Input: dimensioned drawing with shaded views. Units: mm. Origin: part minimum x, y, z. A direction names the side the tool comes from. Coordinates: 2 decimals unless noted, no trailing zeros. Order: outer loops, then holes, each group sorted by start corner. A loop starts at its lowest first (then second) coordinate and runs counter-clockwise, first axis right, second up. Notation, with made-up numbers: (-9.5, -13) - (5.5, -13) arc R25 ccw to (5.5, 20) - close; hole circle Ø5 at (32.5, 29.25). An arc over 180 degrees is marked (long way). One line per question, with ' | ' between items. Start each with the question number.
(1) Section A-A (x = 31.5). Return the cut outline in (y, z), then the cut area to 3 significant figures.
(2) Line query: line 1 along X through (y, z) = (5, 19); line 2 along Z through (x, y) = (62, 10); line 3 along X through (y, z) = (60.5, 26). Output: solid intervals per line, ascending.
(3) Contact query for flat-ended pins moving along their axis: P1, Ø8, axis at x = 10, y = 68.5, coming from the +Z side; P2, Ø12, axis at y = 37.5, z = 19.5, coming from the +X side; P3, Ø17.5, axis at x = 54.5, y = 65.5, coming from the +Z side. Output: stop coordinate, or through.
(4) Access query for the marked faces 1 and 2. Directions: +Z, -Z, +X, -X, +Y, -Y. A direction counts if a zero-diameter tool reaches every point of the face in a straight line with its end or side. Return the directions, or none.
(5) Draft query along Z for the marked faces 3, 4, 5 and 6. Return one class per face: +Z half, -Z half, draft (parallel to the pull), parting line (faces both ways), or undercut.
(6) Section D-D (x = 49). Return the cut outline in (y, z).
(7) Section C-C (z = 20.5). Return the cut outline in (x, y), then the cut area to 3 significant figures.
(8) Section B-B (y = 21). Return the cut outline in (x, z).
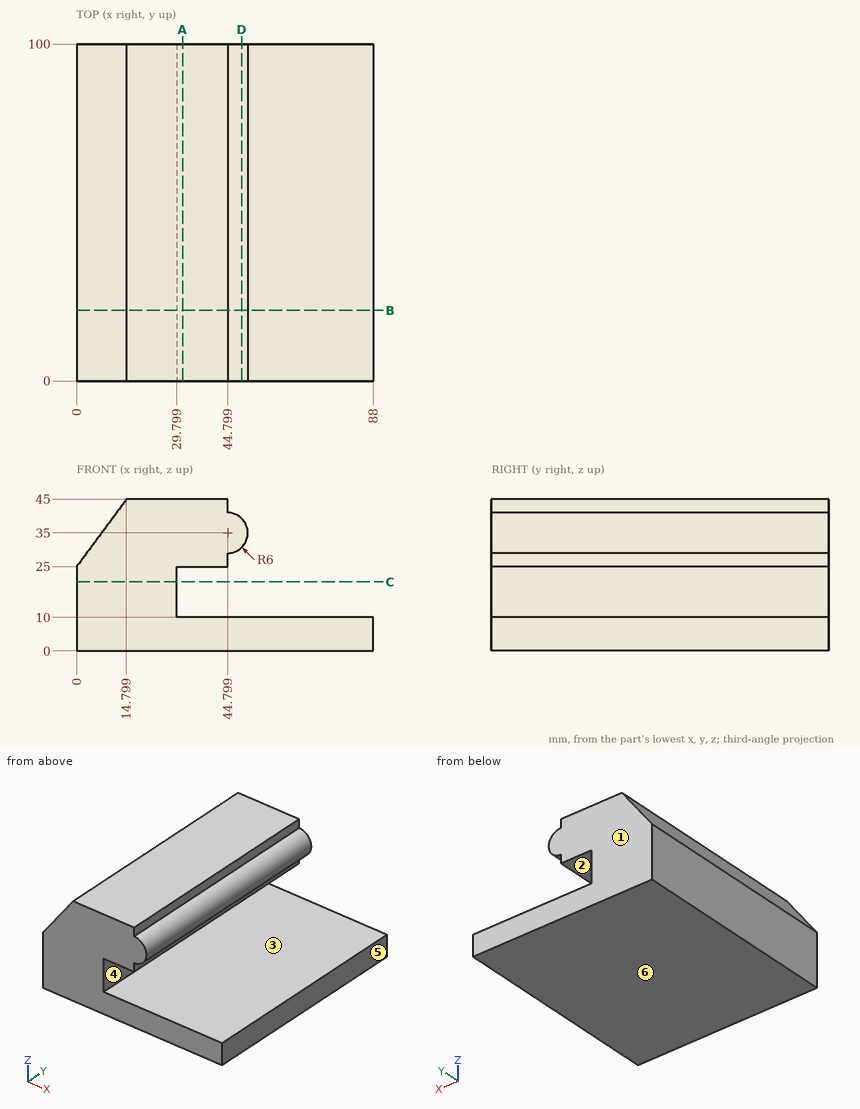
Response values:
1) outline: (0, 0) - (100, 0) - (100, 10) - (0, 10) - close; (0, 25) - (100, 25) - (100, 45) - (0, 45) - close | area: 3,000 mm²
2) line 1: x = 0 to 29.8 | line 2: z = 0 to 10 | line 3: x = 0.74 to 44.8
3) P1: stops at z = 43.92 | P2: stops at x = 44.8 | P3: stops at z = 40.92
4) face 1: +Z, -Z, +X, -X, +Y | face 2: +X, +Y, -Y
5) face 3: undercut | face 4: undercut | face 5: draft | face 6: -Z half
6) outline: (0, 0) - (100, 0) - (100, 10) - (0, 10) - close; (0, 30.72) - (100, 30.72) - (100, 39.28) - (0, 39.28) - close
7) outline: (0, 0) - (29.8, 0) - (29.8, 100) - (0, 100) - close | area: 2,980 mm²
8) outline: (0, 0) - (88, 0) - (88, 10) - (29.8, 10) - (29.8, 25) - (44.8, 25) - (44.8, 29) arc R6 ccw to (50.8, 35) arc R6 ccw to (44.8, 41) - (44.8, 45) - (14.8, 45) - (0, 25) - close
